from build123d import *

# Parameters (mm, degrees)
SKETCH1_W               = 200
SKETCH1_H               = 180
BOSS_EXTRUDE1_DEPTH     = 10
FILLET1_R               = 10
CUT_EXTRUDE5_DEPTH      = 135.907375632
CUT_EXTRUDE5_DEPTH_BACK = 135.907375632
SKETCH26_R              = 1.75
SKETCH27_R              = 3
CUT_EXTRUDE6_DEPTH      = 4
SKETCH28_W              = 70
SKETCH28_H              = 70
BOSS_EXTRUDE2_DEPTH     = 20
CUT_EXTRUDE8_DEPTH      = 138.840487521
CUT_EXTRUDE8_DEPTH_BACK = 138.840487521
FILLET3_R               = 10
FILLET4_R               = 15
CUT_EXTRUDE9_DEPTH      = 137.014705168
CUT_EXTRUDE9_DEPTH_BACK = 137.014705168
SKETCH30_R              = 2.25


with BuildPart() as part:
    # Sketch1 → Boss-Extrude1 (new body)
    with BuildSketch(Plane.XY):
        Rectangle(SKETCH1_W, SKETCH1_H)
    extrude(amount=BOSS_EXTRUDE1_DEPTH)

    # Fillet1
    fillet1_edges = [part.edges().sort_by_distance(p)[0] for p in [
        (100, -90, 5),
        (-100, -90, 5),
        (-100, 90, 5),
        (100, 90, 5),
    ]]
    fillet(fillet1_edges, radius=FILLET1_R)

    # Sketch26 → Cut-Extrude5 (cut, two sides: drawn at the far end of the back side and taken through both)
    with BuildSketch(Plane(origin=(0, 0, 0), x_dir=(-1, 0, 0), z_dir=(0, 0, -1)).offset(-CUT_EXTRUDE5_DEPTH_BACK)):
        with Locations((-79.85, 70)):
            Circle(SKETCH26_R)
        with Locations((-79.85, -70)):
            Circle(SKETCH26_R)
        with Locations((79.85, -70)):
            Circle(SKETCH26_R)
        with Locations((79.85, 70)):
            Circle(SKETCH26_R)
    extrude(amount=CUT_EXTRUDE5_DEPTH + CUT_EXTRUDE5_DEPTH_BACK, mode=Mode.SUBTRACT)

    # Sketch27 → Cut-Extrude6 (cut)
    with BuildSketch(Plane.XY.offset(10)):
        with Locations((-79.85, 70)):
            Circle(SKETCH27_R)
        with Locations((79.85, 70)):
            Circle(SKETCH27_R)
        with Locations((79.85, -70)):
            Circle(SKETCH27_R)
        with Locations((-79.85, -70)):
            Circle(SKETCH27_R)
    extrude(amount=-CUT_EXTRUDE6_DEPTH, mode=Mode.SUBTRACT)

    # Sketch28 → Boss-Extrude2 (add)
    with BuildSketch(Plane.XY.offset(10)):
        with Locations((0, 55)):
            Rectangle(SKETCH28_W, SKETCH28_H)
    extrude(amount=BOSS_EXTRUDE2_DEPTH)

    # Sketch29 → Cut-Extrude8 (cut, two sides: drawn at the far end of the back side and taken through both)
    with BuildSketch(Plane.XY.offset(30).offset(-CUT_EXTRUDE8_DEPTH_BACK)):
        with BuildLine():
            Line((-16.5, 55), (-16.5, 90))
            Line((-16.5, 90), (16.5, 90))
            Line((16.5, 90), (16.5, 55))
            ThreePointArc((16.5, 55), (0, 38.5), (-16.5, 55))
        make_face()
    extrude(amount=CUT_EXTRUDE8_DEPTH + CUT_EXTRUDE8_DEPTH_BACK, mode=Mode.SUBTRACT)

    # Fillet3
    fillet3_edges = [part.edges().sort_by_distance(p)[0] for p in [
        (0, 20, 30),
        (-35, 20, 20),
        (0, 20, 10),
        (-35, 55, 30),
        (-35, 55, 10),
        (35, 55, 30),
        (35, 20, 20),
        (35, 55, 10),
    ]]
    fillet(fillet3_edges, radius=FILLET3_R - 0.0001)  # a hair under: the kernel refuses the full size

    # Fillet4
    fillet4_edges = [part.edges().sort_by_distance(p)[0] for p in [
        (16.5, 90, 15),
        (-16.5, 90, 15),
    ]]
    fillet(fillet4_edges, radius=FILLET4_R)

    # Sketch30 → Cut-Extrude9 (cut, two sides: drawn at the far end of the back side and taken through both)
    with BuildSketch(Plane.XY.offset(10).offset(-CUT_EXTRUDE9_DEPTH_BACK)):
        with Locations((-21.650635095, -67.5)):
            Circle(SKETCH30_R)
        with Locations((21.650635095, -67.5)):
            Circle(SKETCH30_R)
        with Locations((0, -30)):
            Circle(SKETCH30_R)
        with Locations((-79.150635095, -22.5)):
            Circle(SKETCH30_R)
        with Locations((-35.849364905, -22.5)):
            Circle(SKETCH30_R)
        with Locations((-57.5, 15)):
            Circle(SKETCH30_R)
        with Locations((35.849364905, -22.5)):
            Circle(SKETCH30_R)
        with Locations((79.150635095, -22.5)):
            Circle(SKETCH30_R)
        with Locations((57.5, 15)):
            Circle(SKETCH30_R)
    extrude(amount=CUT_EXTRUDE9_DEPTH + CUT_EXTRUDE9_DEPTH_BACK, mode=Mode.SUBTRACT)


solid = part.part
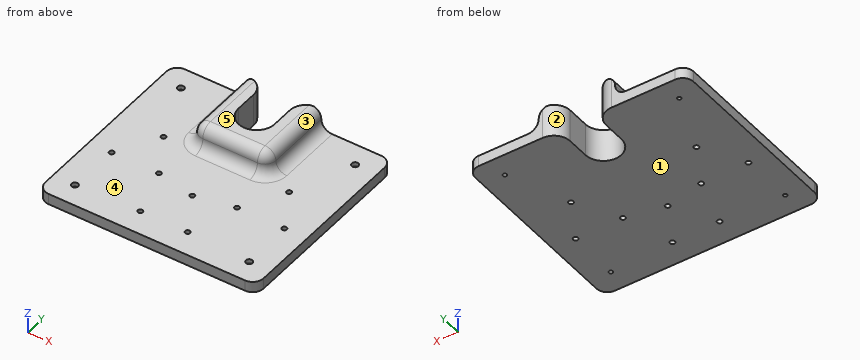
CAD build for the part. Positions are in the model's coordinates, mm. Face numbers are marked on the shaded views. A direction names the side the tool comes from. Round coordinates to 2 decimals unless told otherwise and drop trailing zeros. Write each loop counter-clockwise with the first axis right and the second up, starting at its lowest first coordinate (ties: lowest second). Pieces come first, ordered by that corner, then holes. Notation, with made-up numbers: (11.25, 44) -> (66.25, 44) arc R29 ccw to (66.25, 66) -> close; hole circle Ø6 at (9.5, -29.5). An arc over 180 degrees is marked (long way). Answer as a JSON object with one key per item and string values.
(1) Band-saw the part on C-C, the plane y = -22.5. List the corners of the cut face in (x, z).
Reported:
{"outline": "(-100, 0) -> (-81.4, 0) -> (-81.4, 10) -> (-100, 10) -> close; (-76.9, 0) -> (-38.1, 0) -> (-38.1, 10) -> (-76.9, 10) -> close; (-33.6, 0) -> (33.6, 0) -> (33.6, 10) -> (-33.6, 10) -> close; (38.1, 0) -> (76.9, 0) -> (76.9, 10) -> (38.1, 10) -> close; (81.4, 0) -> (100, 0) -> (100, 10) -> (81.4, 10) -> close"}
(2) Pin check, flat tips, straight feed: P1, Ø3, axis at x = -79.85, y = 70, coming from the -Z side; P2, Ø5, axis at x = 79.85, y = 70, coming from the +Z side; P3, Ø7, axis at x = -79.85, y = -70, coming from the -Z side; P4, Ø1.5, axis at x = 61, y = -6, coming from the +Z side. Stop position of each tip, or through.
Reported:
{"P1": "passes through", "P2": "stops at z = 6", "P3": "stops at z = 0", "P4": "stops at z = 10"}
(3) Probe probe 1 along Y at (x, z) = (-57.5, 5); probe 2 along X at (y, z) = (-22.5, 3.25); probe 3 along X at (y, z) = (15, 2). List the from-to ranges inside material, lowest first. Write a range as [from, to].
Reported:
{"probe 1": "y = [-90, 12.75], [17.25, 90]", "probe 2": "x = [-100, -81.4], [-76.9, -38.1], [-33.6, 33.6], [38.1, 76.9], [81.4, 100]", "probe 3": "x = [-100, -59.75], [-55.25, 55.25], [59.75, 100]"}
(4) Two-plate mould, pull along X, no slides. Class the marked faces 1, 2 and 3: +X half, -X half, draft (parallel to the pull), parting line (faces both ways), or undercut.
Reported:
{"face 1": "draft", "face 2": "undercut", "face 3": "+X half"}
(5) Band-saw the part on D-D, the plane x = -57.5. List the corners of the cut face in (y, z), then the cut area to 4 significant figures.
Reported:
{"outline": "(-90, 0) -> (12.75, 0) -> (12.75, 10) -> (-90, 10) -> close; (17.25, 0) -> (90, 0) -> (90, 10) -> (17.25, 10) -> close", "area": "1,755 mm^2"}
(6) Which spindle directions (+Z, -Z, +X, -X, +Y, -Y) get a long thin tool onto all of the face, cutting with end or side? Do the marked faces 4 and 5. Say none if no direction does.
Reported:
{"face 4": "+Z, -Y", "face 5": "+Z, +X, -X, +Y, -Y"}
